The listing builds one solid part. Answer for the finished solid, in the listing's coordinates (mm). Face numbers are marked on the shaded views. Round coordinates to 2 decimals unless told otherwise and drop trailing zeros. Order: outer loops, then holes, each group sorted by start corner. A loop starts at its lowest first (then second) coordinate and runs counter-clockwise, first axis right, second up. Notation, with made-up numbers: (70, 51) - (121, 51) arc R31 cw to (121, 83) - close; hole circle Ø2 at (-11, 67). An arc over 180 degrees is marked (long way). One line per item, written item: value. Start each with the question number.
1. Section A-A, the plane y = 0 is taken. Give the vertices of the cut face in (x, z).
2. Section C-C, the plane z = 4.5 is taken. Give the vertices of the cut face in (x, y) (1 decimal), then the cut area to 3 significant figures.
3. Straight lines are drawn through the part: line 1 (Y direction, x = 0, z = 8); line 2 (Y direction, x = 0, z = 19.75); line 3 (X direction, y = 0.25, z = 16). For each, find the intervals that lie inside material, in ascending order.
4. Flat-ended cylindrical pins translate along their axes: P1, Ø1, axis at x = -3.5, z = 21, coming from the +Y side; P2, Ø1.7, axis at x = 0, y = -0.5, coming from the +Z side; P3, Ø1.5, axis at y = -2, z = 21.5, coming from the +X side. Find the tip coordinate at first contact, or state that the pin passes through.
5. For a pull along Y with two mould halves and no side action, classify the marked faces 1, 2 and 3 as released by +Y, released by -Y, zero draft, split by the parting line, or undercut.
6. Section B-B, the plane x = 0 is taken. Give the vertices of the cut face in (y, z), then the cut area to 3 significant figures.
7. Section D-D, the plane x = -1.25 is taken. Give the vertices of the cut face in (y, z), then the cut area to 3 significant figures.
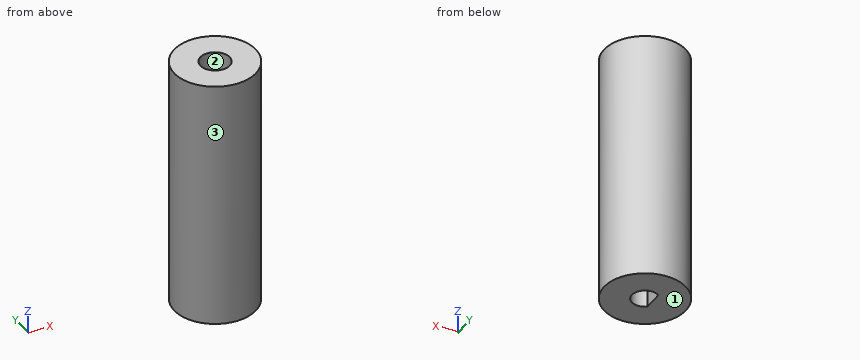
Autodesk Inventor part; units mm, degrees
ref_plane "YZ Plane" through (0, 0, 0) normal (1, 0, 0) x (0, 1, 0)
ref_plane "XZ Plane" through (0, 0, 0) normal (0, 1, 0) x (-1, 0, 0)
ref_plane "XY Plane" through (0, 0, 0) normal (0, 0, 1) x (1, 0, 0)
sketch "Sketch1" plane through (0, 0, 0) normal (0, 0, 1) x (1, 0, 0)
  arc A0 (-0.9144, -1.2192) -> (-0.9144, 1.2192) centre (0, 0) ccw
  line L0 (-0.9144, 1.2192) -> (-0.9144, -1.2192)
  circle A1 centre (0, 0) radius 4.7625
  point P0 (-0.889, 0)
  point P1 (1.524, 0)
  dimension "d0" = 3.048
  dimension "d2" = 2.413
  dimension "d3" = 9.525
extrude "Extrusion1" add sketch "Sketch1" along normal blind 10.16
sketch "Sketch2" plane through (0, 0, 10.16) normal (0, 0, 1) x (1, 0, 0)
  circle A0 centre (0, 0) radius 4.7625
extrude "Extrusion2" add sketch "Sketch2" along normal blind 6.35
sketch "Sketch3" plane through (0, 0, 16.51) normal (0, 0, 1) x (1, 0, 0)
  circle A0 centre (0, 0) radius 4.7625
  circle A1 centre (0, 0) radius 1.7145
  dimension "d8" = 3.429
extrude "Extrusion3" add sketch "Sketch3" along normal blind 12.7
properties part number "Coupling Bushing" material "ABS Plastic"
Answer list:
1. outline: (-4.76, 0) - (-0.91, 0) - (-0.91, 10.16) - (1.52, 10.16) - (1.52, 0) - (4.76, 0) - (4.76, 29.21) - (1.71, 29.21) - (1.71, 16.51) - (-1.71, 16.51) - (-1.71, 29.21) - (-4.76, 29.21) - close
2. outline: circle Ø9.5 at (0, 0); hole (-0.9, -1.2) arc R1.5 ccw (long way) to (-0.9, 1.2) - close
2. area: 65.0 mm²
3. line 1: y = -4.76 to -1.52, 1.52 to 4.76
3. line 2: y = -4.76 to -1.71, 1.71 to 4.76
3. line 3: x = -4.76 to 4.76
4. P1: stops at y = 3.7
4. P2: stops at z = 16.51
4. P3: stops at x = 4.6
5. face 1: zero draft
5. face 2: undercut
5. face 3: split by the parting line
6. outline: (-4.76, 0) - (-1.52, 0) - (-1.52, 10.16) - (1.52, 10.16) - (1.52, 0) - (4.76, 0) - (4.76, 29.21) - (1.71, 29.21) - (1.71, 16.51) - (-1.71, 16.51) - (-1.71, 29.21) - (-4.76, 29.21) - close
6. area: 204 mm²
7. outline: (-4.6, 0) - (4.6, 0) - (4.6, 29.21) - (1.17, 29.21) - (1.17, 16.51) - (-1.17, 16.51) - (-1.17, 29.21) - (-4.6, 29.21) - close
7. area: 239 mm²
